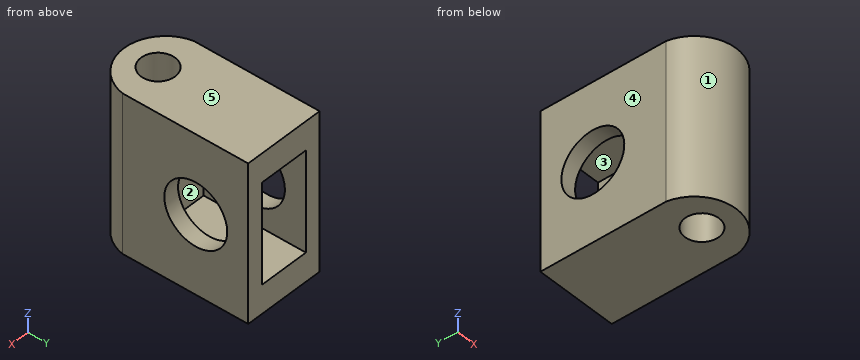
from build123d import *

# Parameters (mm, degrees)
BOSS_EXTRUDE1_DEPTH      = 15
BOSS_EXTRUDE1_DEPTH_BACK = 15
SKETCH1_R                = 3.2385
CUT_EXTRUDE1_START       = -3
SKETCH2_W                = 19.1
SKETCH2_H                = 19.5
CUT_EXTRUDE1_DEPTH       = 9.6
CUT_EXTRUDE2_DEPTH       = 33.316559223
CUT_EXTRUDE2_DEPTH_BACK  = 33.316559223
SKETCH3_R                = 6


with BuildPart() as part:
    # Sketch1 → Boss-Extrude1 (new, two sides: drawn at the far end of the back side and taken through both)
    with BuildSketch(Plane.XY.offset(-BOSS_EXTRUDE1_DEPTH_BACK)):
        with BuildLine():
            Line((-7.8, 0), (-7.8, 24))
            Line((-7.8, 24), (7.8, 24))
            Line((7.8, 24), (7.8, 0))
            ThreePointArc((7.8, 0), (0, -6.5), (-7.8, 0))
        make_face()
        Circle(SKETCH1_R, mode=Mode.SUBTRACT)
    extrude(amount=BOSS_EXTRUDE1_DEPTH + BOSS_EXTRUDE1_DEPTH_BACK)

    # Sketch2 → Cut-Extrude1 (cut)
    with BuildSketch(Plane.ZY.offset(7.8).offset(CUT_EXTRUDE1_START)):
        with Locations((0, 14.25)):
            Rectangle(SKETCH2_W, SKETCH2_H)
    extrude(amount=-CUT_EXTRUDE1_DEPTH, mode=Mode.SUBTRACT)

    # Sketch3 → Cut-Extrude2 (cut, two sides: drawn at the far end of the back side and taken through both)
    with BuildSketch(Plane.ZY.offset(7.8).offset(-CUT_EXTRUDE2_DEPTH_BACK)):
        with Locations((0, 14)):
            Circle(SKETCH3_R)
    extrude(amount=CUT_EXTRUDE2_DEPTH + CUT_EXTRUDE2_DEPTH_BACK, mode=Mode.SUBTRACT)


solid = part.part
The model under review builds one solid part; all positions refer to its coordinate system, in mm. Face numbers are marked on the shaded views. A direction names the side the tool comes from. Give positions to 0.01 mm unless a question says otherwise; leave off trailing zeros. Write each loop counter-clockwise with the first axis right and the second up, starting at its lowest first coordinate (ties: lowest second). Pieces come first, ordered by that corner, then holes.
1. Wall thickness on L1, parallel to X at y = 20, z = 5.5; L2, parallel to Z at x = 3.25, y = 22; L3, parallel to Z at x = -6.85, y = 14: over which ranges is each line inside the solid? List them lowest first.
2. For P1, Ø15.5, axis at y = 14, z = 0, coming from the +X side; P2, Ø1.5, axis at x = 2.5, z = 5.5, coming from the +Y side, all flat-tipped, find the tip position at first contact; note any pin that passes through.
3. Add section D-D, the plane z = 11.5. Write out the cut boundary in (x, y).
4. Add section C-C, the plane x = 0. Write out the cut boundary in (y, z), plus the area to 3 significant figures.
5. Tool access review of the marked faces 1 and 2: name each direction out of +Z, -Z, +X, -X, +Y, -Y from which nothing blocks a thin tool from reaching the whole face with its end or side.
6. Draft analysis for pull direction Z (two halves, no side actions). For the marked faces 3, 4 and 5, state which applies: +Z half, -Z half, draft (parallel to the pull), parting line (faces both ways), or undercut.
7. Add section A-A, the plane z = 0. Write out the cut boundary in (x, y).
8. Add section B-B, the plane y = 14. Write out the cut boundary in (x, z).
Worked answers:
1. L1: x = -7.8 to -4.8, 4.8 to 7.8
1. L2: z = -15 to -9.55, 9.55 to 15
1. L3: z = -15 to -6, 6 to 15
2. P1: stops at x = 7.8
2. P2: stops at y = 4.5
3. outline: (-7.8, 0) arc R7.93 ccw to (7.8, 0) - (7.8, 24) - (-7.8, 24) - close; hole circle Ø6.48 at (0, 0)
4. outline: (-6.5, -15) - (-3.24, -15) - (-3.24, 15) - (-6.5, 15) - close; (3.24, -15) - (24, -15) - (24, -9.55) - (4.5, -9.55) - (4.5, 9.55) - (24, 9.55) - (24, 15) - (3.24, 15) - close
4. area: 348 mm2
5. face 1: +Z, -Z, -Y
5. face 2: +Y
6. face 3: undercut
6. face 4: draft
6. face 5: +Z half
7. outline: (-7.8, 0) arc R7.93 ccw to (7.8, 0) - (7.8, 8) - (4.8, 8) - (4.8, 4.5) - (-4.8, 4.5) - (-4.8, 8) - (-7.8, 8) - close; (-7.8, 20) - (-4.8, 20) - (-4.8, 24) - (-7.8, 24) - close; (4.8, 20) - (7.8, 20) - (7.8, 24) - (4.8, 24) - close; hole circle Ø6.48 at (0, 0)
8. outline: (-7.8, -15) - (7.8, -15) - (7.8, -6) - (4.8, -6) - (4.8, -9.55) - (-4.8, -9.55) - (-4.8, -6) - (-7.8, -6) - close; (-7.8, 6) - (-4.8, 6) - (-4.8, 9.55) - (4.8, 9.55) - (4.8, 6) - (7.8, 6) - (7.8, 15) - (-7.8, 15) - close
